Job drawing, mm, ordinate dimensions from the low corner. One solid piece. Round coordinates to 2 decimals unless told otherwise and drop trailing zeros. Write each loop counter-clockwise with the first axis right and the second up, starting at its lowest first coordinate (ties: lowest second). Pieces come first, ordered by that corner, then holes.
1) Flat gauge pins, fed straight in: pin 1 (6 mm diameter, centred on x = 33, y = 18.5, fed in from +Z); pin 2 (5 mm diameter, centred on y = 14.5, z = 34.5, fed in from +X); pin 3 (10 mm diameter, centred on y = 39, z = 58, fed in from +X). Where does each tip first touch, or does it go through?
2) Wall check: probe 1 along Y at (x, z) = (50, 76); probe 2 along Y at (x, z) = (50, 16); probe 3 along Z at (x, y) = (65.5, 24). Give the ranges that are in metal, low to high.
3) Saw through at B-B (x = 50). Write the cut outline in (y, z), plus the area to 3 significant figures.
4) Pull direction X, two halves, no side cores. Call the marked faces 1, 2 and 3: +X half, -X half, draft (parallel to the pull), parting line (faces both ways), or undercut.
5) Saw through at A-A (z = 87). Write the cut outline in (x, y), plus the area to 3 significant figures.
6) Saw through at C-C (z = 17). Write the cut outline in (x, y).
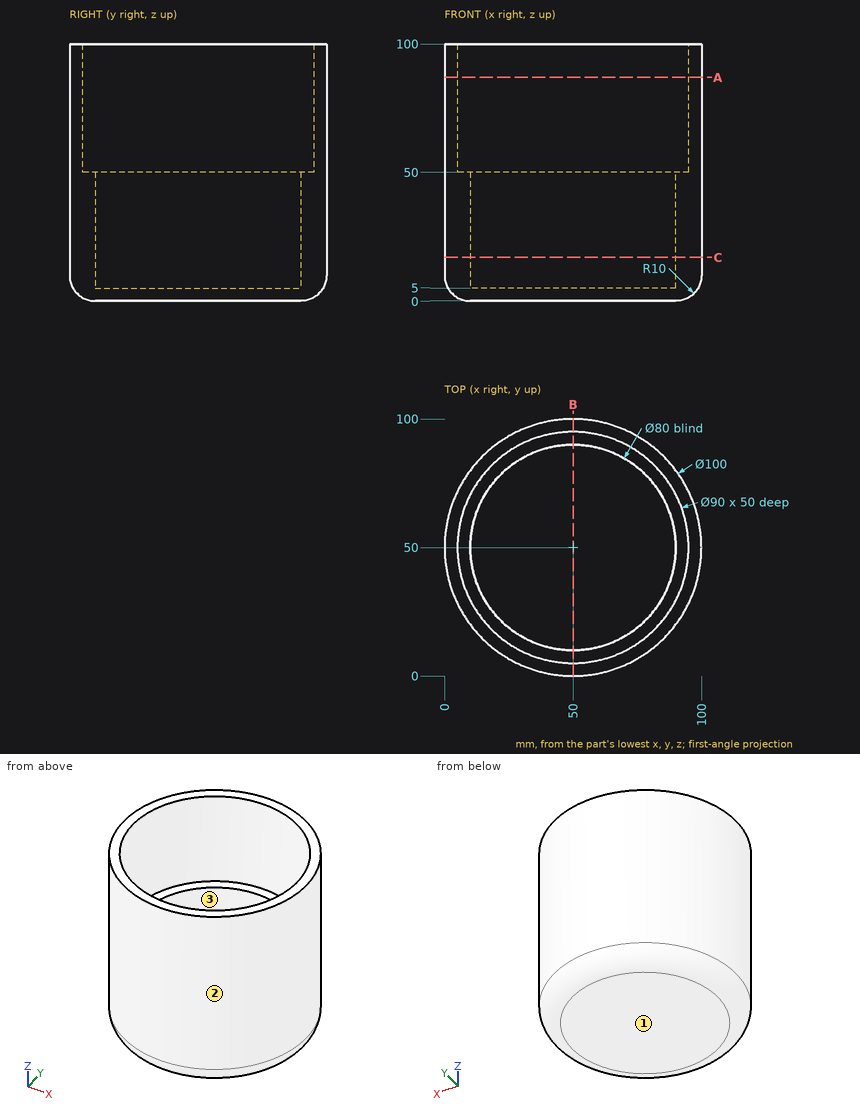
Evaluation:
1. pin 1: stops at z = 5
1. pin 2: stops at x = 87.56
1. pin 3: stops at x = 99.64
2. probe 1: y = 0 to 5, 95 to 100
2. probe 2: y = 0 to 10, 90 to 100
2. probe 3: z = 0 to 5
3. outline: (0, 10) arc R10 ccw to (10, 0) - (90, 0) arc R10 ccw to (100, 10) - (100, 100) - (95, 100) - (95, 50) - (90, 50) - (90, 5) - (10, 5) - (10, 50) - (5, 50) - (5, 100) - (0, 100) - close
3. area: 1,860 mm2
4. face 1: draft
4. face 2: parting line
4. face 3: undercut
5. outline: circle Ø100 at (50, 50); hole circle Ø90 at (50, 50)
5. area: 1,490 mm2
6. outline: circle Ø100 at (50, 50); hole circle Ø80 at (50, 50)
